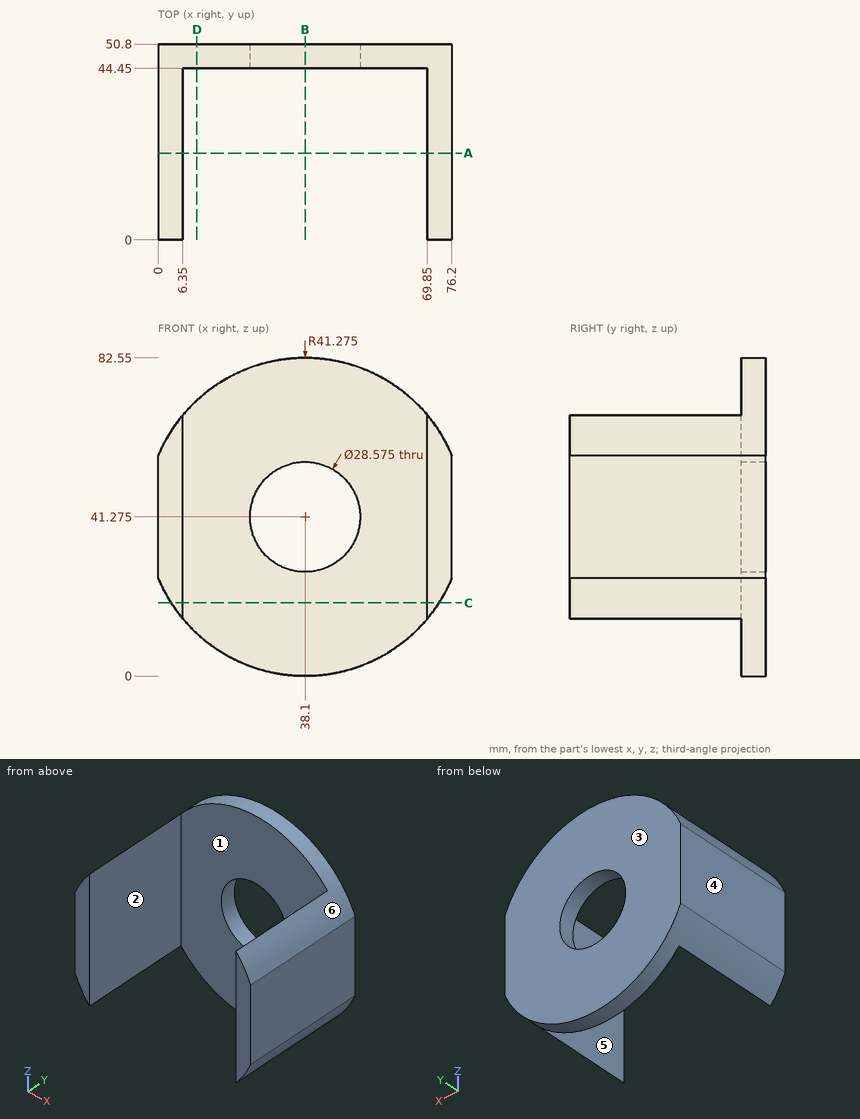
Check sheet for the drawn part. Datum: minimum x, y, z corner. Units: mm. A direction names the side the tool comes from. Coordinates: 2 decimals unless noted, no trailing zeros. Write each loop counter-clockwise with the first axis right and the second up, starting at its lowest first coordinate (ties: lowest second). Pieces come first, ordered by that corner, then holes. Notation, with made-up numbers: M -13.75,-7.75 L 18.25,-7.75 A14 cw 18.25,16.25 Z; hole C 50,32 d1. An arc over 180 degrees is marked long. Use a Markdown table: item, result.
Q1. Sectioned sample at A-A, the plane y = 22.5. Record the boundary of the cut face in (x, z) (3 decimals).
Reply:
| item | result |
|---|---|
| outline | M 0,25.4 A41.275 ccw 6.35,14.901 L 6.35,67.649 A41.275 ccw 0,57.15 Z; M 69.85,14.901 A41.275 ccw 76.2,25.4 L 76.2,57.15 A41.275 ccw 69.85,67.649 Z |
Q2. Sectioned sample at C-C, the plane z = 19. Record the boundary of the cut face in (x, y), plus the area to 3 significant figures.
Reply:
| item | result |
|---|---|
| outline | M 3.35,0 L 6.35,0 L 6.35,44.45 L 69.85,44.45 L 69.85,0 L 72.85,0 L 72.85,50.8 L 3.35,50.8 Z |
| area | 708 mm² |
Q3. Thickness scan on line 1 (Z direction, x = 38, y = 47); line 2 (X direction, y = 22, z = 27). Record the ranges inside material, lowest first.
Reply:
| item | result |
|---|---|
| line 1 | z = 0 to 26.99, 55.56 to 82.55 |
| line 2 | x = 0 to 6.35, 69.85 to 76.2 |
Q4. Set-up check for the marked faces 5 and 6: record each of +Z, -Z, +X, -X, +Y, -Y from which the full face is reachable in a straight line by a thin tool's end or side.
Reply:
| item | result |
|---|---|
| face 5 | +Z, -Z, -Y |
| face 6 | +Z, +Y, -Y |
Q5. Draft check along X on the marked faces 1, 2, 3 and 4. Enter one of: +X half, -X half, draft (parallel to the pull), parting line (faces both ways), or undercut.
Reply:
| item | result |
|---|---|
| face 1 | undercut |
| face 2 | undercut |
| face 3 | draft |
| face 4 | -X half |
Q6. Sectioned sample at D-D, the plane x = 10. Record the boundary of the cut face in (y, z).
Reply:
| item | result |
|---|---|
| outline | M 44.45,11.04 L 50.8,11.04 L 50.8,71.51 L 44.45,71.51 Z |
Q7. Sectioned sample at B-B, the plane x = 38.1. Record the boundary of the cut face in (y, z), plus the area to 3 significant figures.
Reply:
| item | result |
|---|---|
| outline | M 44.45,0 L 50.8,0 L 50.8,26.99 L 44.45,26.99 Z; M 44.45,55.56 L 50.8,55.56 L 50.8,82.55 L 44.45,82.55 Z |
| area | 343 mm² |
Q8. Go/stop test with flat-tipped pins: P1, Ø5, axis at y = 16, z = 19.5, coming from the -X side; P2, Ø2, axis at x = 24, z = 66.5, coming from the -Y side. Record where each tip stops, or that it passes through.
Reply:
| item | result |
|---|---|
| P1 | stops at x = 1.6 |
| P2 | stops at y = 44.45 |
